Check sheet for the modelled part. Datum: model origin and axes. Units: mm. Coordinates: 2 decimals unless noted, no trailing zeros. Write each loop counter-clockwise with the first axis right and the second up, starting at its lowest first coordinate (ties: lowest second). Pieces come first, ordered by that corner, then holes. Notation, with made-up numbers: (-8, 12) -> (2, 12) arc R13 ccw to (2, 21) -> close; hole circle Ø7 at (19, 48.5). An arc over 180 degrees is marked (long way). Put each result on its own line as item: value.
```python
from build123d import *

# Parameters (mm, degrees)
SALIENTE_EXTRUIR1_DEPTH = 3
CROQUIS2_R              = 67.5
CROQUIS2_R_2            = 2.25
CROQUIS2_R_3            = 1.6
CORTAR_EXTRUIR1_DEPTH   = 3


with BuildPart() as part:
    # Croquis1 → Saliente-Extruir1 (new body)
    with BuildSketch(Plane.XY):
        Polygon((-261.838674033, 298.703267526), (-260.838674033, 298.703267526), (-260.838674033, 323.703267526), (187.161325967, 323.703267526), (187.161325967, 298.703267526), (188.161325967, 298.703267526), (188.161325967, -197.096732474), (-261.838674033, -197.096732474), align=None)
    extrude(amount=SALIENTE_EXTRUIR1_DEPTH)

    # Croquis2 → Cortar-Extruir1 (cut)
    with BuildSketch(Plane.XY.offset(3)):
        with Locations((-114.838674033, -29.596732474)):
            Circle(CROQUIS2_R)
        with Locations((-52.588674033, 32.653267526)):
            Circle(CROQUIS2_R_2)
        with Locations((-34.838674033, 50.403267526)):
            Circle(CROQUIS2_R_3)
        with Locations((-52.588674033, -91.846732474)):
            Circle(CROQUIS2_R_2)
        with Locations((-34.838674033, -109.596732474)):
            Circle(CROQUIS2_R_3)
        with Locations((-177.088674033, -91.846732474)):
            Circle(CROQUIS2_R_2)
        with Locations((-194.838674033, -109.596732474)):
            Circle(CROQUIS2_R_3)
        with Locations((-177.088674033, 32.653267526)):
            Circle(CROQUIS2_R_2)
        with Locations((-194.838674033, 50.403267526)):
            Circle(CROQUIS2_R_3)
    extrude(amount=-CORTAR_EXTRUIR1_DEPTH, mode=Mode.SUBTRACT)


solid = part.part
```
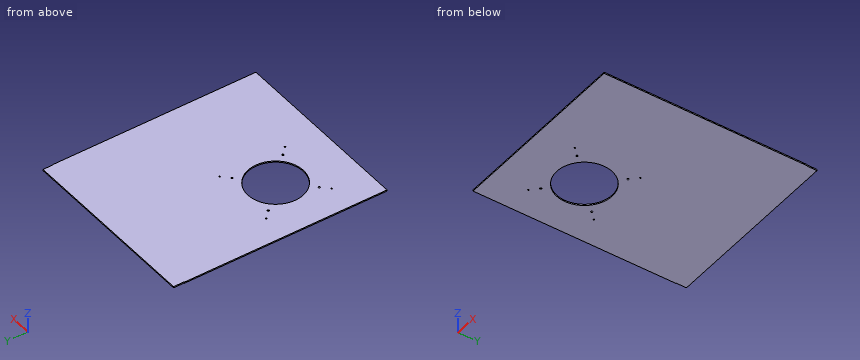
Q1. Cross-section at B-B (x = -135). Record the cut outline in (y, z).
Recorded:
outline: (-197.1, 0) -> (-94.02, 0) -> (-94.02, 3) -> (-197.1, 3) -> close; (34.82, 0) -> (323.7, 0) -> (323.7, 3) -> (34.82, 3) -> close
Q2. Material ranges on line 1 along X through (y, z) = (24, 2.6); line 2 along Y through (x, z) = (-60, 0.3); line 3 along X through (y, z) = (-42, 0.35), recorded low to high.
Recorded:
line 1: x = -261.84 to -155.87, -73.81 to 188.16
line 2: y = -197.1 to -68.95, 9.76 to 323.7
line 3: x = -261.84 to -181.19, -48.49 to 188.16
Q3. Cross-section at A-A (y = -1). Record the cut outline in (x, z), plus the area to 3 significant figures.
Recorded:
outline: (-261.84, 0) -> (-175.98, 0) -> (-175.98, 3) -> (-261.84, 3) -> close; (-53.7, 0) -> (188.16, 0) -> (188.16, 3) -> (-53.7, 3) -> close
area: 983 mm2
Q4. Depth check by flat-ended pin: P1, Ø7, axis at x = -52.59, y = -91.85, coming from the -Z side; P2, Ø0.5, axis at x = 187.5, z = 1.5, coming from the +Y side. Enter the tip coordinate at first touch or a pass-through.
Recorded:
P1: stops at z = 0
P2: stops at y = 298.7
Q5. Cross-section at C-C (z = 1). State how many separate pieces and enclosed holes the cut face has, plus the area to 3 significant figures.
Recorded:
separate pieces: 1
enclosed holes: 9
area: 220,000 mm2
